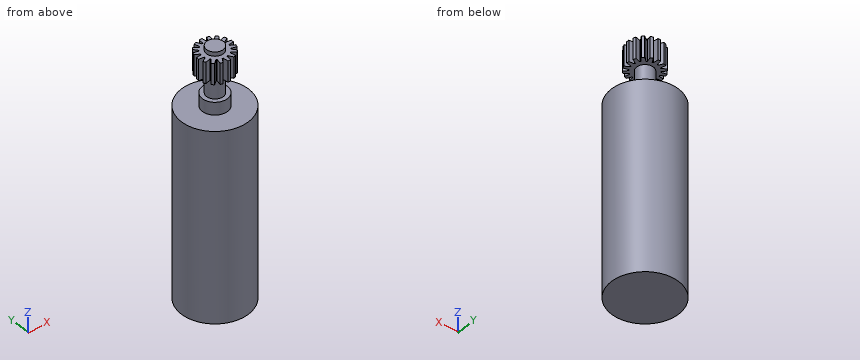
from build123d import *

# Parameters (mm, degrees)
ESBO_O1_R                = 8
RESSALTO_EXTRUS_O1_DEPTH = 45
ESBO_O2_R                = 3
RESSALTO_EXTRUS_O2_DEPTH = 3
ESBO_O3_R                = 2
RESSALTO_EXTRUS_O3_DEPTH = 5
ESBO_O4_R                = 3
RESSALTO_EXTRUS_O4_DEPTH = 5
ESBO_O5_R                = 2
RESSALTO_EXTRUS_O5_DEPTH = 1
RESSALTO_EXTRUS_O6_DEPTH = 5
PADR_OCIRCULAR1_COUNT    = 16


with BuildPart() as part:
    # Esboço1 → Ressalto-extrusão1 (new body)
    with BuildSketch(Plane.XY):
        Circle(ESBO_O1_R)
    extrude(amount=RESSALTO_EXTRUS_O1_DEPTH)

    # Esboço2 → Ressalto-extrusão2 (add)
    with BuildSketch(Plane.XY.offset(45)):
        Circle(ESBO_O2_R)
    extrude(amount=RESSALTO_EXTRUS_O2_DEPTH)

    # Esboço3 → Ressalto-extrusão3 (add)
    with BuildSketch(Plane.XY.offset(48)):
        Circle(ESBO_O3_R)
    extrude(amount=RESSALTO_EXTRUS_O3_DEPTH)

    # Esboço4 → Ressalto-extrusão4 (add)
    with BuildSketch(Plane.XY.offset(53)):
        Circle(ESBO_O4_R)
    extrude(amount=RESSALTO_EXTRUS_O4_DEPTH)

    # Esboço5 → Ressalto-extrusão5 (add)
    with BuildSketch(Plane.XY.offset(58)):
        Circle(ESBO_O5_R)
    extrude(amount=RESSALTO_EXTRUS_O5_DEPTH)

    # Esboço6 → Ressalto-extrusão6 (add)
    with BuildSketch(Plane.XY.offset(58)):
        Polygon((-0.5, 2.735669954), (-0.317294901, 4.179040235), (0.317294901, 4.179040235), (0.5, 2.735669954), align=None)
    ressalto_extrus_o6 = extrude(amount=-RESSALTO_EXTRUS_O6_DEPTH)

    # PadrãoCircular1: Ressalto-extrusão6 ×16 about axis
    padr_ocircular1_axis = Axis((0, 0, 0), (0, 0, 1))
    for i in range(1, PADR_OCIRCULAR1_COUNT):
        add(ressalto_extrus_o6.rotate(padr_ocircular1_axis, i * 360 / PADR_OCIRCULAR1_COUNT))


solid = part.part
Part model, mm, in its own coordinate system. Coordinates: 2 decimals unless noted, no trailing zeros. Order: outer loops, then holes, each group sorted by start corner. A loop starts at its lowest first (then second) coordinate and runs counter-clockwise, first axis right, second up. Notation, with made-up numbers: M -29.5,47 L -0.5,47 A22 cw -0.5,59 Z; hole C -20.5,-12 d10. An arc over 180 degrees is marked long. Use a Markdown table: item, result.
(1) Cut at B-B on z = 22. Write the cut outline in (x, y), then the cut area to 3 significant figures.
A:
| item | result |
|---|---|
| outline | C 0,0 d16 |
| area | 201 mm^2 |
(2) Flat gauge pins, fed straight in: pin 1 (4 mm diameter, centred on x = 2.5, z = 36, fed in from +Y); pin 2 (0.7 mm diameter, centred on y = 0, z = 56, fed in from -X); pin 3 (3 mm diameter, centred on x = 5.5, y = 0.5, fed in from +Z). Where does each tip first touch, or does it go through?
A:
| item | result |
|---|---|
| pin 1 | stops at y = 7.98 |
| pin 2 | stops at x = -4.18 |
| pin 3 | stops at z = 58 |
(3) Probe L1, parallel to Z at x = 1.75, y = 2.25; L2, parallel to Y at x = 2.5, z = 55; L3, parallel to Z at x = 1, y = 5. List the from-to ranges inside material, lowest first.
A:
| item | result |
|---|---|
| L1 | z = 0 to 48, 53 to 58 |
| L2 | y = -3 to -1.85, -1.66 to 1.66, 1.85 to 3 |
| L3 | z = 0 to 45 |
(4) Cut at A-A on y = -6.5. Write the cut outline in (x, z).
A:
| item | result |
|---|---|
| outline | M -4.66,0 L 4.66,0 L 4.66,45 L -4.66,45 Z |
